Can you work these out from the drawing? Everything is in mm from the part's minimum corner. Round coordinates to 2 decimals unless told otherwise and drop trailing zeros. Write each loop counter-clockwise with the first axis right and the second up, starting at its lowest first coordinate (ties: lowest second). Pieces come first, ordered by that corner, then holes. Notation, with made-up numbers: M -28.75,34 L -0.75,34 A13 ccw -0.75,46 Z; hole C 19.25,65 d6. An arc over 180 degrees is marked long. Answer in a Markdown table with one row per item. Add a question column.
(1) Suppose I cut it at A-A, the plane x = 81. Write out the boundary of the cut face in (y, z).
(2) I'm going to push flat-ended pins straight in: pin 1 (3 mm diameter, centred on x = 164, y = 96, fed in from +Z); pin 2 (3 mm diameter, centred on x = 199, z = 105, fed in from +Y); pin 3 (5 mm diameter, centred on x = 66.5, y = 14, fed in from -Z); pin 4 (11 mm diameter, centred on x = 135.5, z = 107.5, fed in from -Y). Where does each tip first touch, or does it pass through?
(3) If I drill on probe 1 along Y at (x, z) = (197.5, 105); probe 2 along Z at (x, y) = (41.5, 43), over which ranges is the centre line in solid material (lowest first)?
(4) If we mould it in two halves opening along Y, with no side actions, what happens to the marked faces 1, 2 and 3? For each: released by +Y, released by -Y, zero draft, split by the parting line, or undercut.
(5) Suppose I cut it at B-B, the plane y = 41. Write out the boundary of the cut face in (x, z).
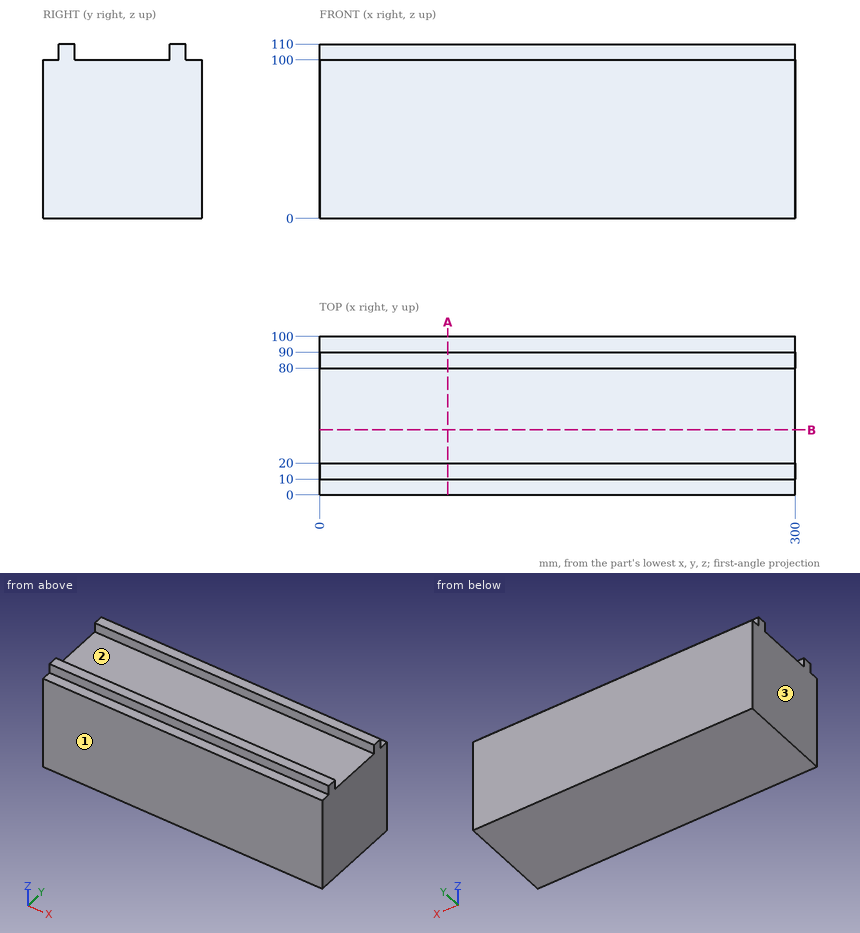
Calculated:
| question | item | result |
|---|---|---|
| 1 | outline | M 0,0 L 100,0 L 100,100 L 90,100 L 90,110 L 80,110 L 80,100 L 20,100 L 20,110 L 10,110 L 10,100 L 0,100 Z |
| 2 | pin 1 | z = 100 |
| 2 | pin 2 | y = 90 |
| 2 | pin 3 | z = 0 |
| 2 | pin 4 | y = 10 |
| 3 | probe 1 | 10 to 20, 80 to 90 |
| 3 | probe 2 | 0 to 100 |
| 4 | face 1 | released by -Y |
| 4 | face 2 | undercut |
| 4 | face 3 | zero draft |
| 5 | outline | M 0,0 L 300,0 L 300,100 L 0,100 Z |
